from build123d import *

# Parameters (mm, degrees)
SKETCH1_W           = 76.2
SKETCH1_H           = 76.2
SKETCH1_R           = 8.73125
SKETCH1_R_2         = 5.55625
BOSS_EXTRUDE1_DEPTH = 9.525
CUT_EXTRUDE1_DEPTH  = 6.604
SKETCH1_3_R         = 5.55625
BOSS_EXTRUDE2_DEPTH = 12.7


with BuildPart() as part:
    # Sketch1 → Boss-Extrude1 (new body)
    # profile 1 of 2: a face of its own
    with BuildSketch(Plane(origin=(0, 0, 0), x_dir=(1, 0, 0), z_dir=(0, 1, 0))):
        Rectangle(SKETCH1_W, SKETCH1_H)
        with Locations(Location((0, 0, 0), (0, 0, 90))):
            Circle(SKETCH1_R, mode=Mode.SUBTRACT)
        with Locations(Location((-26.9875, -26.9875, 0), (0, 0, 90))):
            Circle(SKETCH1_R_2, mode=Mode.SUBTRACT)
        with Locations(Location((26.9875, -26.9875, 0), (0, 0, 90))):
            Circle(SKETCH1_R_2, mode=Mode.SUBTRACT)
        with Locations((26.9875, 26.9875)):
            Circle(SKETCH1_R_2, mode=Mode.SUBTRACT)
        with Locations(Location((-26.9875, 26.9875, 0), (0, 0, 90))):
            Circle(SKETCH1_R_2, mode=Mode.SUBTRACT)
    # profile 2 of 2: a face of its own
    with BuildSketch(Plane(origin=(0, 0, 0), x_dir=(1, 0, 0), z_dir=(0, 1, 0))):
        with Locations((26.9875, 26.9875)):
            Circle(SKETCH1_R_2)
    extrude(amount=BOSS_EXTRUDE1_DEPTH)

    # Sketch2 → Cut-Extrude1 (cut)
    with BuildSketch(Plane(origin=(0, 9.525, 0), x_dir=(1, 0, 0), z_dir=(0, 1, 0))):
        Polygon((-38.1, -9.525), (-8.73125, 0), (0, -8.73125), (-9.525, -38.1), (-38.1, -38.1), align=None)
    extrude(amount=-CUT_EXTRUDE1_DEPTH, mode=Mode.SUBTRACT)

    # Sketch1_3 → Boss-Extrude2 (add)
    with BuildSketch(Plane(origin=(0, 0, 0), x_dir=(1, 0, 0), z_dir=(0, 1, 0))):
        with Locations(Location((26.9875, 26.9875, 0), (0, 0, 270))):
            Circle(SKETCH1_3_R)
    extrude(amount=BOSS_EXTRUDE2_DEPTH)


solid = part.part
Build history of the part. All positions in model axes, mm. A direction names the side the tool comes from. Coordinates: 2 decimals unless noted, no trailing zeros. Order: outer loops, then holes, each group sorted by start corner. A loop starts at its lowest first (then second) coordinate and runs counter-clockwise, first axis right, second up. Notation, with made-up numbers: (19, 13.25) -> (43, 13.25) arc R17 cw to (43, 44.25) -> close; hole circle Ø9 at (-15.5, -9.5). An arc over 180 degrees is marked (long way). One line per item, written item: value.
(1) Slice it at B-B, the plane x = 30.5. List the corners of the cut face in (y, z) (3 decimals).
Checked values:
outline: (0, -38.1) -> (9.525, -38.1) -> (9.525, -31.293) -> (12.7, -31.293) -> (12.7, -22.682) -> (9.525, -22.682) -> (9.525, 22.682) -> (0, 22.682) -> close; (0, 31.293) -> (9.525, 31.293) -> (9.525, 38.1) -> (0, 38.1) -> close
(2) Slice it at D-D, the plane x = 19.5. List the corners of the cut face in (y, z) (3 decimals).
Checked values:
outline: (0, -38.1) -> (9.525, -38.1) -> (9.525, 38.1) -> (0, 38.1) -> close
(3) Slice it at A-A, the plane z = -23. List the corners of the cut face in (x, y) (3 decimals), plus the area to 3 significant figures.
Checked values:
outline: (-38.1, 0) -> (-30.857, 0) -> (-30.857, 9.525) -> (-38.1, 9.525) -> close; (-23.118, 0) -> (38.1, 0) -> (38.1, 9.525) -> (30.857, 9.525) -> (30.857, 12.7) -> (23.118, 12.7) -> (23.118, 9.525) -> (-23.118, 9.525) -> close
area: 677 mm2
(4) Tool access for faces 1 (the cylindrical face through (24.859, 11.09, -21.855)), 2 (the flat face through (9, 0, -1)): list every direction of +Z, -Z, +X, -X, +Y, -Y with a clear straight run to the whole face (end or side of a thin tool).
Checked values:
face 1: +Y
face 2: +Z, -Z, +X, -X, -Y
(5) Slice it at C-C, the plane y = 4.75. List the corners of the cut face in (x, z) (1 decimal).
Checked values:
outline: (-38.1, -38.1) -> (38.1, -38.1) -> (38.1, 38.1) -> (-9.5, 38.1) -> (0, 8.7) arc R8.7 cw (long way) to (-8.7, 0) -> (-38.1, 9.5) -> close; hole circle Ø11.1 at (-27, -27); hole circle Ø11.1 at (27, 27)
(6) Probe line 1 (X direction, y = 2.5, z = 0); line 2 (Z direction, x = -26, y = 0.5); line 3 (X direction, y = 2.5, z = 2.5). List the from-to ranges inside material, lowest first. Write a range as [from, to].
Checked values:
line 1: [-38.1, -8.73], [8.73, 38.1]
line 2: [-38.1, -32.46], [-21.52, 21.52], [32.46, 38.1]
line 3: [-38.1, -8.37], [8.37, 38.1]
(7) Drop flat-ended pins along their axis: pin 1 Ø1.5 at (x, z) = (-27, 30) entering from -Y; pin 2 Ø14.5 at (x, z) = (26.99, 26.99) entering from +Y (3 decimals). Give the stop position or say it passes through.
Checked values:
pin 1: through
pin 2: y = 9.525
(8) Mould opens along X. For faces 3 (the cylindrical face through (3.344, 4.696, -8.065)), 4 (the flat face through (8, 9.525, -9)), 5 (the cylindrical face through (-21.563, 4.696, -25.783)), 6 (the flat face through (-38.1, 5, -8)) say: pulls with the +X half, pulls with the -X half, needs draft (parallel to the pull), parting line crosses it, or undercut.
Checked values:
face 3: undercut
face 4: needs draft
face 5: undercut
face 6: pulls with the -X half
